Read the model definition and answer for the solid it produces. Units are mm, in the model's axes. A direction names the side the tool comes from. Coordinates: 2 decimals unless noted, no trailing zeros. Order: outer loops, then holes, each group sorted by start corner. A loop starts at its lowest first (then second) coordinate and runs counter-clockwise, first axis right, second up. Notation, with made-up numbers: M 18,45 L 42,45 A26 cw 42,75 Z; hole C 23,-6.5 d8. An arc over 180 degrees is marked long. Use a Markdown table: item, result. Add a question column.
1) Find section C-C on y = 41.5. Write down the section's boundary in (x, z).
2) Each of these flat-tipped pins is pushed along its axis until it touches: pin 1 Ø9 at (x, z) = (51, 43) entering from +Y; pin 2 Ø1 at (y, z) = (36.5, 13.5) entering from +X; pin 3 Ø8 at (x, z) = (45.5, 14.5) entering from +Y. Where does it stop, or does it pass through?
3) Find section B-B on z = 27.5. Write down the section's boundary in (x, y).
4) Find the intervals of material crossed by probe 1 along Y at (x, z) = (53, 40); probe 2 along X at (y, z) = (34.5, 49.5), in increasing order. Write a range as [from, to].
5) For faces 1 (the face through (23, 23, 60)), 2 (the face through (15, 45, 45)), determine the directions among +Z, -Z, +X, -X, +Y, -Y from which every point of the face is accessible in a straight line to the end or side of a thin tool.
6) Find section A-A on x = 42.5. Write down the section's boundary in (y, z), plus the area to 4 significant figures.
7) Find section D-D on z = 55.5. Write down the section's boundary in (x, y).
from build123d import *

# Parameters (mm, degrees)
CROQUIS1_W              = 60
CROQUIS1_H              = 60
SALIENTE_EXTRUIR1_DEPTH = 60
CROQUIS2_W              = 30
CROQUIS2_H              = 30
CORTAR_EXTRUIR1_DEPTH   = 30
CORTAR_EXTRUIR2_DEPTH   = 30
CORTAR_EXTRUIR3_DEPTH   = 30


with BuildPart() as part:
    # Croquis1 → Saliente-Extruir1 (new body)
    with BuildSketch(Plane(origin=(0, 0, 0), x_dir=(1, 0, 0), z_dir=(0, 1, 0))):
        with Locations((30, -30)):
            Rectangle(CROQUIS1_W, CROQUIS1_H)
    extrude(amount=SALIENTE_EXTRUIR1_DEPTH)

    # Croquis2 → Cortar-Extruir1 (cut)
    with BuildSketch(Plane(origin=(0, 60, 0), x_dir=(1, 0, 0), z_dir=(0, 1, 0))):
        with Locations((45, -45)):
            Rectangle(CROQUIS2_W, CROQUIS2_H)
    extrude(amount=-CORTAR_EXTRUIR1_DEPTH, mode=Mode.SUBTRACT)

    # Croquis3 → Cortar-Extruir2 (cut)
    with BuildSketch(Plane.XY.offset(30)):
        Polygon((30, 60), (60, 30), (60, 60), align=None)
    extrude(amount=-CORTAR_EXTRUIR2_DEPTH, mode=Mode.SUBTRACT)

    # Croquis4 → Cortar-Extruir3 (cut)
    with BuildSketch(Plane.XY.offset(60)):
        Polygon((0, 60), (30, 30), (30, 60), align=None)
    extrude(amount=-CORTAR_EXTRUIR3_DEPTH, mode=Mode.SUBTRACT)


solid = part.part
Check result:
| question | item | result |
|---|---|---|
| 1 | outline | M 0,0 L 48.5,0 L 48.5,30 L 18.5,30 L 18.5,60 L 0,60 Z |
| 2 | pin 1 | stops at y = 30 |
| 2 | pin 2 | stops at x = 54 |
| 2 | pin 3 | stops at y = 48.5 |
| 3 | outline | M 0,0 L 60,0 L 60,30 L 30,60 L 0,60 Z |
| 4 | probe 1 | y = [0, 30] |
| 4 | probe 2 | x = [0, 25.5] |
| 5 | face 1 | +Z, +X, -X, +Y, -Y |
| 5 | face 2 | +Z, +X, +Y |
| 6 | outline | M 0,0 L 47.5,0 L 47.5,30 L 30,30 L 30,60 L 0,60 Z |
| 6 | area | 2,325 mm2 |
| 7 | outline | M 0,0 L 60,0 L 60,30 L 30,30 L 0,60 Z |
